Source: CAD feature listing. Evaluate the final solid. Frame: model axes, mm. A direction names the side the tool comes from. Give positions to 0.01 mm unless a question says otherwise; leave off trailing zeros. Order: outer loops, then holes, each group sorted by start corner. A loop starts at its lowest first (then second) coordinate and runs counter-clockwise, first axis right, second up. Notation, with made-up numbers: (72.5, 11.25) - (92.5, 11.25) arc R25 cw to (92.5, 43.25) - close; hole circle Ø5 at (24, 51.5). An arc over 180 degrees is marked (long way). Use CSV: the item, a comma, the result in double quotes.
```python
from build123d import *

# Parameters (mm, degrees)
F1_DEPTH = 30.48
F2_W     = 10.7188
F2_H     = 6.1722
F3_DEPTH = 6.35
F4_W     = 10.16
F4_H     = 5.08
F5_DEPTH = 25.4
F7_DEPTH = 30.48


with BuildPart() as f1:
    # F0 (on Front) → F1 (new body)
    with BuildSketch(Plane.XZ):
        Polygon((76.2921414277, 0), (-76.1078585723, 0), (-55.7878585723, -15.24), (55.9721414277, -15.24), align=None)
    extrude(amount=F1_DEPTH)

    # F2 (on face) → F3 (cut)
    with BuildSketch(Plane.XY):
        with Locations((0, -15.24)):
            Rectangle(F2_W, F2_H)
    extrude(amount=-F3_DEPTH, mode=Mode.SUBTRACT)

    # F4 (on face) → F5 (cut)
    with BuildSketch(Plane.XZ.offset(12.1539)):
        with Locations((0, -3.297025953)):
            Rectangle(F4_W, F4_H)
    extrude(amount=-F5_DEPTH, mode=Mode.SUBTRACT)

    # F6 (on face) → F7 (join)
    with BuildSketch(Plane(origin=(0, 0, 0), x_dir=(-1, 0, 0), z_dir=(0, 1, 0))):
        Polygon((62.3605558789, -10.31047702), (55.7878585723, -15.24), (65.9478585723, -15.24), (71.7585558789, -10.31047702), align=None)
        Polygon((-55.9721414277, -15.24), (-62.5448387344, -10.31047702), (-71.9428387344, -10.31047702), (-66.1321414277, -15.24), align=None)
    extrude(amount=-F7_DEPTH)


solid = f1.part
```
Item 1: First-contact query: pin 1 (1 mm diameter, centred on y = -4, z = -11.5, fed in from -X); pin 2 (4 mm diameter, centred on y = -10.5, z = -8, fed in from -X); pin 3 (2 mm diameter, centred on y = -24, z = -2, fed in from +X). Flat tips, straight axial feed; report the tip coordinate or a pass-through.
Filled in:
pin 1,"stops at x = -70.95"
pin 2,"stops at x = -68.11"
pin 3,"stops at x = 74.96"
Item 2: Material intervals for line 1 (X direction, y = -18, z = -3.25); line 2 (X direction, y = -5, z = -4.5); line 3 (Y direction, x = -4, z = -2), sorted ascending. Write a range as from..to.
Filled in:
line 1,"x = -71.77..-5.36, 5.36..71.96"
line 2,"x = -70.11..-5.08, 5.08..70.29"
line 3,"y = -30.48..-18.33"
Item 3: Section D-D on x = -64. Return the cut outline in (y, z), then the cut area to 3 significant figures.
Filled in:
outline,"(-30.48, -15.24) - (0, -15.24) - (0, -10.31) - (-30.48, -10.31) - close; (-30.48, -9.08) - (0, -9.08) - (0, 0) - (-30.48, 0) - close"
area,"427 mm2"
Item 4: Mould query, pull axis Y, two halves, no side actions, for faces 4 (the flat face through (-69.33, -15.027, -5.083)), 5 (the flat face through (1, -30.48, -8)), 6 (the flat face through (5.359, -15, -3)). Classes: released by +Y, released by -Y, zero draft, split by the parting line, or undercut.
Filled in:
face 4,"zero draft"
face 5,"released by -Y"
face 6,"undercut"
Item 5: Section B-B on y = -3. Return the cut outline in (x, z), then the cut area to 3 significant figures.
Filled in:
outline,"(-76.11, 0) - (-62.36, -10.31) - (-71.76, -10.31) - (-65.95, -15.24) - (66.13, -15.24) - (71.94, -10.31) - (62.54, -10.31) - (76.29, 0) - close; hole (-5.08, -5.84) - (5.08, -5.84) - (5.08, -0.76) - (-5.08, -0.76) - close"
area,"2,060 mm2"
Item 6: Set-up query: faces 1 (the flat face through (1, -12, 0)), 2 (the flat face through (5.08, -6, -3)), 3 (the flat face through (0, -15, -6.35)). Return all of +Z, -Z, +X, -X, +Y, -Y with unobstructed straight access to the full face (end or side cutting, diameter ignored); none if empty.
Filled in:
face 1,"+Z, +X, -X, +Y, -Y"
face 2,"+Y"
face 3,"+Z"
Item 7: Section C-C on y = -22. Return the cut outline in (x, z), then the cut area to 3 significant figures.
Filled in:
outline,"(-76.11, 0) - (-62.36, -10.31) - (-71.76, -10.31) - (-65.95, -15.24) - (66.13, -15.24) - (71.94, -10.31) - (62.54, -10.31) - (76.29, 0) - close"
area,"2,110 mm2"
Item 8: Section A-A on x = -0.5. Return the cut outline in (y, z), then the cut area to 3 significant figures.
Filled in:
outline,"(-30.48, -15.24) - (0, -15.24) - (0, -5.84) - (-12.15, -5.84) - (-12.15, -6.35) - (-18.33, -6.35) - (-18.33, 0) - (-30.48, 0) - close; (-12.15, -0.76) - (0, -0.76) - (0, 0) - (-12.15, 0) - close"
area,"364 mm2"
